Here's how the part is built. I have some questions about the finished solid (model axes, mm). A direction names the side the tool comes from. Coordinates: 2 decimals unless noted, no trailing zeros. Order: outer loops, then holes, each group sorted by start corner. A loop starts at its lowest first (then second) coordinate and runs counter-clockwise, first axis right, second up. Notation, with made-up numbers: (37.25, 81) - (87.25, 81) arc R37 ccw to (87.25, 120) - close; hole circle Ø4 at (81, -24). An arc over 180 degrees is marked (long way). Answer as CSV lines item,"result". Start each with the question number.
Item 1: We'd pull the mould along X, two halves only. Please class faces 1 (the face through (8, 2.2, 2)), 2 (the face through (2, -2.2, 5.2)), 3 (the face through (4.5, -2.2, 5.2)), 4 (the face through (7.883, 7, 2)): pulls with the +X half, pulls with the -X half, needs draft (parallel to the pull), parting line crosses it, or undercut.
Item 2: Imagine slicing it at C-C on y = 4.2. List the corners of the cut face in (x, z) for me.
Item 3: Imagine slicing it at B-B on y = 23.5. List the corners of the cut face in (x, z) for me, and give its area (3 significant figures).
Item 4: Imagine slicing it at A-A on y = -1.5. List the corners of the cut face in (x, z) for me, and give its area (3 significant figures).
Item 5: Imagine slicing it at D-D on y = 33. List the corners of the cut face in (x, z) for me.
Item 6: I'm going to push flat-ended pins straight in: pin 1 (0.6 mm diameter, centred on y = 14, z = 2, fed in from +X); pin 2 (0.6 mm diameter, centred on y = -1.5, z = 4.5, fed in from -X) (3 decimals); pin 3 (1.6 mm diameter, centred on y = -4.5, z = 4.5, fed in from -X); pin 4 (0.6 mm diameter, centred on x = 15, y = 4.5, fed in from +Z). Where does each tip first touch, or does it pass through?
Item 7: I need wall thicknesses on line 1 (Y direction, x = 7.25, z = 2.4); line 2 (Y direction, x = 4.25, z = 2.4); line 3 (Z direction, x = 6.5, y = 23). Which ranges of each line are inside material? Lowest first, please.
Item 8: On a 3-axis mill with a long thin cutter (end or side, diameter ignored), from which of +Z, -Z, +X, -X, +Y, -Y can I reach the whole of each face in a straight line? I mean faces 5 (the face through (9, -2.2, 5.2)), 6 (the face through (4, 5, 2.5)), 7 (the face through (15.5, 1, 2)), 8 (the face through (5.464, 5, 2)). Say none if no direction works.
from build123d import *

# Parameters (mm, degrees)
SKETCH_1_W                     = 16
SKETCH_1_H                     = 37
EXTRUDE_1_DEPTH                = 1.5
SKETCH_2_W                     = 15
SKETCH_2_H                     = 2
EXTRUDE_2_DEPTH                = 2
SKETCH_3_W                     = 0.5
SKETCH_3_H                     = 0.5
EXTRUDE_3_DEPTH                = 2
SKETCH_4_W                     = 0.5
SKETCH_4_H                     = 0.5
EXTRUDE_4_DEPTH                = 8
FILLET_2_R                     = 0.5
FILLET_3_R                     = 0.2
PATTERN_LINEAR_1_COUNT         = 6
PATTERN_LINEAR_1_PITCH         = 2.5
FILLET_2_OF_PATTERN_LINEAR_1_R = 0.5
FILLET_3_OF_PATTERN_LINEAR_1_R = 0.2
SKETCH_7_W                     = 13
SKETCH_7_H                     = 5.5
EXTRUDE_7_DEPTH                = 0.5
SKETCH_8_W                     = 13
SKETCH_8_H                     = 21.5
EXTRUDE_8_DEPTH                = 0.5
SKETCH_9_W                     = 2
SKETCH_9_H                     = 3
EXTRUDE_9_DEPTH                = 0.8
SKETCH_10_R                    = 0.5
EXTRUDE_10_DEPTH               = 0.5
SKETCH_11_W                    = 2
SKETCH_11_H                    = 1
EXTRUDE_11_DEPTH               = 1
SKETCH_12_W                    = 7
SKETCH_12_H                    = 7
SKETCH_12_W_2                  = 9
SKETCH_12_H_2                  = 6
EXTRUDE_12_DEPTH               = 0.5


with BuildPart() as part:
    # 草图1 → 凸台-拉伸1 (new body)
    with BuildSketch(Plane.XY):
        with Locations((8, 18.5)):
            Rectangle(SKETCH_1_W, SKETCH_1_H)
    extrude(amount=EXTRUDE_1_DEPTH)

    # 草图2 → 凸台-拉伸2 (add)
    with BuildSketch(Plane.XY.offset(1.5)):
        with Locations((8, 1.2)):
            Rectangle(SKETCH_2_W, SKETCH_2_H)
    extrude(amount=EXTRUDE_2_DEPTH)

    # 草图3 → 凸台-拉伸3 (add)
    with BuildSketch(Plane.XY.offset(3.5)):
        with Locations((1.75, 1.2)):
            Rectangle(SKETCH_3_W, SKETCH_3_H)
    extrude_3 = extrude(amount=EXTRUDE_3_DEPTH)

    # 草图4 → 凸台-拉伸4 (add)
    with BuildSketch(Plane.XZ.offset(-0.95)):
        with Locations((1.75, 5.25)):
            Rectangle(SKETCH_4_W, SKETCH_4_H)
    extrude_4 = extrude(amount=EXTRUDE_4_DEPTH)

    # 圆角2
    fillet_2_edges = [part.edges().sort_by_distance(p)[0] for p in [
        (1.75, 1.45, 5.5),
    ]]
    fillet(fillet_2_edges, radius=FILLET_2_R)

    # 圆角3
    fillet_3_edges = [part.edges().sort_by_distance(p)[0] for p in [
        (1.75, 0.95, 5),
    ]]
    fillet(fillet_3_edges, radius=FILLET_3_R)

    # 阵列(线性)1: 凸台-拉伸3, 凸台-拉伸4 ×6
    with Locations(*[(i * PATTERN_LINEAR_1_PITCH, 0, 0) for i in range(1, PATTERN_LINEAR_1_COUNT)]):
        add(extrude_3)
        add(extrude_4)

    # 圆角2 of 阵列(线性)1
    fillet_2_of_pattern_linear_1_edges = [part.edges().sort_by_distance(p)[0] for p in [
        (4.25, 1.45, 5.5),
        (6.75, 1.45, 5.5),
        (9.25, 1.45, 5.5),
        (11.75, 1.45, 5.5),
        (14.25, 1.45, 5.5),
    ]]
    fillet(fillet_2_of_pattern_linear_1_edges, radius=FILLET_2_OF_PATTERN_LINEAR_1_R)

    # 圆角3 of 阵列(线性)1
    fillet_3_of_pattern_linear_1_edges = [part.edges().sort_by_distance(p)[0] for p in [
        (4.25, 0.95, 5),
        (6.75, 0.95, 5),
        (9.25, 0.95, 5),
        (11.75, 0.95, 5),
        (14.25, 0.95, 5),
    ]]
    fillet(fillet_3_of_pattern_linear_1_edges, radius=FILLET_3_OF_PATTERN_LINEAR_1_R)

    # 草图7 → 凸台-拉伸7 (add)
    with BuildSketch(Plane.XY.offset(1.5)):
        with Locations((8, 34.05)):
            Rectangle(SKETCH_7_W, SKETCH_7_H)
    extrude(amount=EXTRUDE_7_DEPTH)

    # 草图8 → 凸台-拉伸8 (add)
    with BuildSketch(Plane.XY.offset(1.5)):
        with Locations((8, 20.45)):
            Rectangle(SKETCH_8_W, SKETCH_8_H)
    extrude(amount=EXTRUDE_8_DEPTH)

    # 草图9 → 凸台-拉伸9 (add)
    with BuildSketch(Plane.XY.offset(1.5)):
        with Locations((14.8, 4.2)):
            Rectangle(SKETCH_9_W, SKETCH_9_H)
    extrude(amount=EXTRUDE_9_DEPTH)

    # 草图10 → 凸台-拉伸10 (add)
    with BuildSketch(Plane.XY.offset(2.3)):
        with Locations((14.8, 4.2)):
            Circle(SKETCH_10_R)
    extrude(amount=EXTRUDE_10_DEPTH)

    # 草图11 → 凸台-拉伸11 (add)
    with BuildSketch(Plane.XY.offset(1.5)):
        with Locations((8.882624218, 7.325014272)):
            Rectangle(SKETCH_11_W, SKETCH_11_H)
        with Locations((4.464220441, 5.288706444)):
            Rectangle(SKETCH_11_W, SKETCH_11_H)
    extrude(amount=EXTRUDE_11_DEPTH)

    # 草图12 → 凸台-拉伸12 (add)
    with BuildSketch(Plane.XY.offset(2)):
        with Locations((10.3, 20.4)):
            Rectangle(SKETCH_12_W, SKETCH_12_H)
        with Locations((9.3, 13.4)):
            Rectangle(SKETCH_12_W_2, SKETCH_12_H_2)
    extrude(amount=EXTRUDE_12_DEPTH)


solid = part.part
Responses:
1,face 1,"needs draft"
1,face 2,"undercut"
1,face 3,"undercut"
1,face 4,"pulls with the -X half"
2,outline,"(0, 0) - (16, 0) - (16, 1.5) - (15.8, 1.5) - (15.8, 2.3) - (15.3, 2.3) - (15.3, 2.8) - (14.3, 2.8) - (14.3, 2.3) - (13.8, 2.3) - (13.8, 1.5) - (0, 1.5) - close"
3,outline,"(0, 0) - (16, 0) - (16, 1.5) - (14.5, 1.5) - (14.5, 2) - (13.8, 2) - (13.8, 2.5) - (6.8, 2.5) - (6.8, 2) - (1.5, 2) - (1.5, 1.5) - (0, 1.5) - close"
3,area,"34.0 mm^2"
4,outline,"(1.5, 5) - (2, 5) - (2, 5.5) - (1.5, 5.5) - close; (4, 5) - (4.5, 5) - (4.5, 5.5) - (4, 5.5) - close; (6.5, 5) - (7, 5) - (7, 5.5) - (6.5, 5.5) - close; (9, 5) - (9.5, 5) - (9.5, 5.5) - (9, 5.5) - close; (11.5, 5) - (12, 5) - (12, 5.5) - (11.5, 5.5) - close; (14, 5) - (14.5, 5) - (14.5, 5.5) - (14, 5.5) - close"
4,area,"1.50 mm^2"
5,outline,"(0, 0) - (16, 0) - (16, 1.5) - (14.5, 1.5) - (14.5, 2) - (1.5, 2) - (1.5, 1.5) - (0, 1.5) - close"
6,pin 1,"stops at x = 14.5"
6,pin 2,"passes through"
6,pin 3,"stops at x = 1.5"
6,pin 4,"stops at z = 2.8"
7,line 1,"y = 0.2 to 2.2, 10.4 to 16.4, 16.9 to 23.9"
7,line 2,"y = 0.2 to 2.2, 4.79 to 5.79"
7,line 3,"z = 0 to 2"
8,face 5,"+Z, +Y, -Y"
8,face 6,"+Z, +X, -X, +Y"
8,face 7,"+Z, +X, -Y"
8,face 8,"+Z"
